The listing builds one solid part. Answer for the finished solid, in the listing's coordinates (mm). Face numbers are marked on the shaded views. A direction names the side the tool comes from. Give positions to 0.01 mm unless a question says otherwise; leave off trailing zeros. Write each loop counter-clockwise with the first axis right and the second up, starting at its lowest first coordinate (ties: lowest second). Pieces come first, ordered by that corner, then holes.
```python
from build123d import *

# Parameters (mm, degrees)
SKETCH1_W           = 65
SKETCH1_H           = 80
BOSS_EXTRUDE1_DEPTH = 15
SKETCH2_R           = 1.75
CUT_EXTRUDE1_DEPTH  = 15
SKETCH3_W           = 6.452545503
SKETCH3_H           = 5.641605939
CUT_EXTRUDE2_DEPTH  = 9
FILLET1_R           = 2
SHELL1_START        = -10
SHELL1_DEPTH        = 10
SHELL1_START_2      = -1
SHELL1_2_DEPTH      = 1
SKETCH4_W           = 31
SKETCH4_H           = 9.988916405
CUT_EXTRUDE3_DEPTH  = 9
SKETCH5_W           = 9.944131197
SKETCH5_H           = 30.964366914
SKETCH5_W_2         = 9.409197356
SKETCH5_H_2         = 30.907117663
CUT_EXTRUDE4_DEPTH  = 9
SKETCH6_W           = 8.400929104
SKETCH6_H           = 4.591319751
SKETCH6_W_2         = 30.7
SKETCH6_H_2         = 9.525851227
CUT_EXTRUDE5_DEPTH  = 9
CUT_EXTRUDE6_DEPTH  = 9


# Read off the part's stored shape, not the designer's step: Shell1
with BuildPart() as part:
    # Sketch1 → Boss-Extrude1 (new body)
    with BuildSketch(Plane.XY):
        with Locations((-32.5, 40)):
            Rectangle(SKETCH1_W, SKETCH1_H)
    extrude(amount=-BOSS_EXTRUDE1_DEPTH)

    # Sketch2 → Cut-Extrude1 (cut)
    with BuildSketch(Plane.XY):
        with Locations((-3, 3)):
            Circle(SKETCH2_R)
        with Locations((-62, 3)):
            Circle(SKETCH2_R)
        with Locations((-62, 77)):
            Circle(SKETCH2_R)
        with Locations((-3, 77)):
            Circle(SKETCH2_R)
    extrude(amount=-CUT_EXTRUDE1_DEPTH, mode=Mode.SUBTRACT)

    # Sketch3 → Cut-Extrude2 (cut)
    with BuildSketch(Plane(origin=(0, 0, -15), x_dir=(-1, 0, 0), z_dir=(0, 0, -1))):
        with Locations((3.226272752, 77.179197031)):
            Rectangle(SKETCH3_W, SKETCH3_H)
        with Locations((61.773727249, 77.179197031)):
            Rectangle(SKETCH3_W, SKETCH3_H)
        with Locations((3.226272752, 2.82080297)):
            Rectangle(SKETCH3_W, SKETCH3_H)
        with Locations((61.773727249, 2.82080297)):
            Rectangle(SKETCH3_W, SKETCH3_H)
    extrude(amount=-CUT_EXTRUDE2_DEPTH, mode=Mode.SUBTRACT)

    # Fillet1
    fillet1_edges = [part.edges().sort_by_distance(p)[0] for p in [
        (-32.5, 0, -15),
        (-65, 40, -15),
        (-32.5, 80, -15),
        (0, 40, -15),
        (-58.547454497, 77.17919703, -15),
        (-61.773727249, 74.358394061, -15),
        (-58.547454497, 74.358394061, -10.5),
        (-58.547454497, 80, -10.5),
        (-65, 74.358394061, -10.5),
        (-6.452545503, 2.82080297, -15),
        (-3.226272751, 5.641605939, -15),
        (0, 5.641605939, -10.5),
        (-6.452545503, 5.641605939, -10.5),
        (-6.452545503, 0, -10.5),
        (-58.547454497, 2.82080297, -15),
        (-61.773727249, 5.641605939, -15),
        (-58.547454497, 0, -10.5),
        (-58.547454497, 5.641605939, -10.5),
        (-65, 5.641605939, -10.5),
        (-3.226272751, 74.358394061, -15),
        (-6.452545503, 77.17919703, -15),
        (0, 74.358394061, -10.5),
        (-6.452545503, 80, -10.5),
        (-6.452545503, 74.358394061, -10.5),
    ]]
    fillet(fillet1_edges, radius=FILLET1_R)

    # Shell1 outline → Shell1 (cut)
    with BuildSketch(Plane.XY.offset(SHELL1_START)):
        with BuildLine():
            ThreePointArc((-11.319478266, 5), (-9.104410686, 8.872299041), (-5, 10.620165502))
            Line((-5, 10.620165502), (-5, 69.379834498))
            ThreePointArc((-5, 69.379834498), (-9.104410686, 71.127700959), (-11.319478266, 75))
            Line((-11.319478266, 75), (-53.680521734, 75))
            ThreePointArc((-53.680521734, 75), (-55.895589314, 71.127700959), (-60, 69.379834498))
            Line((-60, 69.379834498), (-60, 10.620165502))
            ThreePointArc((-60, 10.620165502), (-55.895589314, 8.872299041), (-53.680521734, 5))
            Line((-53.680521734, 5), (-11.319478266, 5))
        make_face()
    extrude(amount=SHELL1_DEPTH, mode=Mode.SUBTRACT)

    # Shell1 2 outline → Shell1 2 (cut)
    with BuildSketch(Plane.XY.offset(SHELL1_START_2)):
        with BuildLine():
            ThreePointArc((-9.446898479, 5), (-7.772970773, 7.772970773), (-5, 9.446898479))
            Line((-5, 9.446898479), (-5, 10.620165502))
            ThreePointArc((-5, 10.620165502), (-9.104410686, 8.872299041), (-11.319478266, 5))
            Line((-11.319478266, 5), (-9.446898479, 5))
        make_face()
        with BuildLine():
            ThreePointArc((-11.319478266, 75), (-9.104410686, 71.127700959), (-5, 69.379834498))
            Line((-5, 69.379834498), (-5, 70.553101521))
            ThreePointArc((-5, 70.553101521), (-7.772970773, 72.227029227), (-9.446898479, 75))
            Line((-9.446898479, 75), (-11.319478266, 75))
        make_face()
        with BuildLine():
            Line((-55.553101521, 5), (-53.680521734, 5))
            ThreePointArc((-53.680521734, 5), (-55.895589314, 8.872299041), (-60, 10.620165502))
            Line((-60, 10.620165502), (-60, 9.446898479))
            ThreePointArc((-60, 9.446898479), (-57.227029227, 7.772970773), (-55.553101521, 5))
        make_face()
        with BuildLine():
            ThreePointArc((-60, 69.379834498), (-55.895589314, 71.127700959), (-53.680521734, 75))
            Line((-53.680521734, 75), (-55.553101521, 75))
            ThreePointArc((-55.553101521, 75), (-57.227029227, 72.227029227), (-60, 70.553101521))
            Line((-60, 70.553101521), (-60, 69.379834498))
        make_face()
    extrude(amount=SHELL1_2_DEPTH, mode=Mode.SUBTRACT)

    # Sketch4 → Cut-Extrude3 (cut)
    with BuildSketch(Plane.XZ):
        with Locations((-24.8, -4.994458203)):
            Rectangle(SKETCH4_W, SKETCH4_H)
    extrude(amount=-CUT_EXTRUDE3_DEPTH, mode=Mode.SUBTRACT)

    # Sketch5 → Cut-Extrude4 (cut)
    with BuildSketch(Plane(origin=(0, 0, 0), x_dir=(0, 0, -1), z_dir=(1, 0, 0))):
        with Locations((4.972065599, 57.356572465)):
            Rectangle(SKETCH5_W, SKETCH5_H)
        with Locations((4.704598678, 23.640694869)):
            Rectangle(SKETCH5_W_2, SKETCH5_H_2)
    extrude(amount=-CUT_EXTRUDE4_DEPTH, mode=Mode.SUBTRACT)

    # Sketch6 → Cut-Extrude5 (cut)
    with BuildSketch(Plane(origin=(0, 80, 0), x_dir=(1, 0, 0), z_dir=(0, 1, 0))):
        with Locations((-48.526627408, 2.295659876)):
            Rectangle(SKETCH6_W, SKETCH6_H)
        with Locations((-24.643720135, 4.762925614)):
            Rectangle(SKETCH6_W_2, SKETCH6_H_2)
    extrude(amount=-CUT_EXTRUDE5_DEPTH, mode=Mode.SUBTRACT)

    # Sketch7 → Cut-Extrude6 (cut)
    with BuildSketch(Plane.ZY.offset(65)):
        Polygon((-0.41148, 7.238999939), (0, 7.238999939), (0, 68.347517032), (-0.41148, 68.347517032), (-9.049681563, 68.347517032), (-9.049681563, 7.238999939), align=None)
    extrude(amount=-CUT_EXTRUDE6_DEPTH, mode=Mode.SUBTRACT)


solid = part.part
```
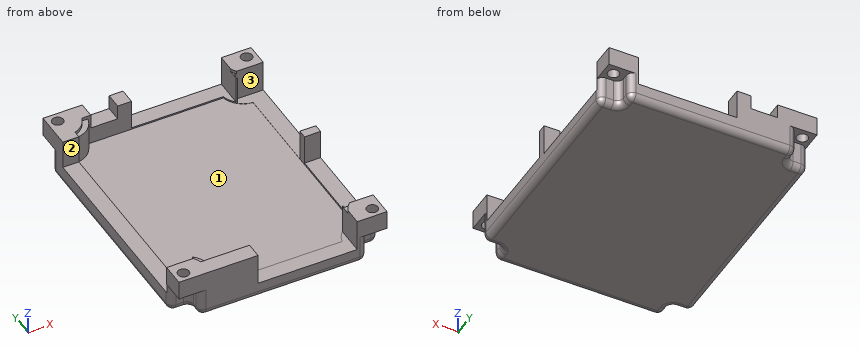
Item 1: A cutting plane is placed at D-D, the plane y = 23. Give the vertices of the cut face in (x, z), plus the area to 3 significant figures.
Conclusion:
outline: (-65, -13) arc R2 ccw to (-63, -15) - (-2, -15) arc R2 ccw to (0, -13) - (0, -9.41) - (-5, -9.41) - (-5, -10) - (-60, -10) - (-60, -9.05) - (-65, -9.05) - close
area: 331 mm2
Item 2: Which of the six approach directions +Z, -Z, +X, -X, +Y, -Y give full straight-line access (tool end or side, diameter ignored) to the marked faces 1, 2 and 3?
Conclusion:
face 1: +Z
face 2: +Z, +X, -X
face 3: +Z, +X
Item 3: Each of these flat-tipped pins is pushed along its axis until it touches: P1, Ø0.8, axis at y = 3, z = -11, coming from the +X side; P2, Ø2.5, axis at x = -59, y = 29.5, coming from the +Z side; P3, Ø0.6, axis at x = -9, y = 8, coming from the +Z side. Where does it stop, or does it pass through?
Conclusion:
P1: stops at x = -6.45
P2: stops at z = -9.05
P3: stops at z = -1
Item 4: A cutting plane is placed at A-A, the plane x = -3. Give the vertices of the cut face in (y, z).
Conclusion:
outline: (0, -6) - (1.25, -6) - (1.25, 0) - (0, 0) - close; (4.75, -6) - (5.64, -6) - (5.64, -13) arc R2 ccw to (7.64, -15) - (72.36, -15) arc R2 ccw to (74.36, -13) - (74.36, -6) - (75.25, -6) - (75.25, 0) - (72.84, 0) - (72.84, -9.94) - (41.87, -9.94) - (41.87, 0) - (39.09, 0) - (39.09, -9.41) - (8.19, -9.41) - (8.19, 0) - (4.75, 0) - close; (78.75, -6) - (80, -6) - (80, 0) - (78.75, 0) - close
Item 5: Consider probe 1 along Y at (x, z) = (-3, -4.25); probe 2 along X at (y, z) = (77, -4.35); probe 3 along Y at (x, z) = (-40.5, -6). Determine where each line is inside the solid, lowest interval first.
Conclusion:
probe 1: y = 0 to 1.25, 4.75 to 8.19, 39.09 to 41.87, 72.84 to 75.25, 78.75 to 80
probe 2: x = -65 to -63.75, -60.25 to -52.73, -44.33 to -39.99, -9.29 to -4.75, -1.25 to 0
probe 3: y = 0 to 5, 75 to 80
Item 6: A cutting plane is placed at B-B, the plane z = -2.75. Count the separate pieces of the cut face and the enclosed holes in it, plus the area to 3 significant figures.
Conclusion:
separate pieces: 6
enclosed holes: 4
area: 410 mm2
